Autodesk Inventor part; units mm, degrees
ref_plane "YZ Plane" through (0, 0, 0) normal (1, 0, 0) x (0, 1, 0)
ref_plane "XZ Plane" through (0, 0, 0) normal (0, 1, 0) x (-1, 0, 0)
ref_plane "XY Plane" through (0, 0, 0) normal (0, 0, 1) x (1, 0, 0)
sketch "Sketch1" plane through (0, 0, 0) normal (0, 1, 0) x (-1, 0, 0)
  line L0 (-100, 325) -> (100, 325)
  line L1 (100, 325) -> (100, -325)
  line L2 (100, -325) -> (-100, -325)
  line L3 (-100, -325) -> (-100, 325)
  line L4 (-100, 325) -> (100, -325) construction
  line L5 (100, 325) -> (-100, -325) construction
  point P0 (0, 0)
  dimension "d0" = 200
  dimension "d1" = 650
sketch "Sketch2" plane through (0, 0, 0) normal (0, 1, 0) x (-1, 0, 0)
  point P0 (0, 0)
extrude "Extrusion1" add sketch "Sketch1" along normal blind 20
sketch "Sketch3" plane through (0, 20, 0) normal (0, 1, 0) x (1, 0, 0)
  line L0 (-100, -325) -> (100, -325)
  arc A0 (-100, -325) -> (91.7903, -325) centre (-4.1048, -57.5933) ccw
  point P0 (0, 0)
extrude "Extrusion2" add sketch "Sketch3" against normal blind 20
sketch "Sketch4" plane through (0, 20, 0) normal (0, 1, 0) x (1, 0, 0)
  line L0 (100, 325) -> (-100, 325)
  line L1 (100, 325) -> (36.9346, 362.619)
  line L2 (36.9346, 362.619) -> (0, 367.9885)
  line L3 (0, 367.9885) -> (-39.4325, 362.619)
  line L4 (-39.4325, 362.619) -> (-100, 325)
  point P0 (0, 0)
extrude "Extrusion3" add sketch "Sketch4" against normal blind 20
fillet "Fillet1" radius 2 1 edges at (100, 10, 325)
fillet "Fillet2" radius 4 1 edges at (-100, 10, 325)
chamfer "Chamfer1" distance 2 angle 45 1 edges at (0, 10, -367.9885)
fillet "Fillet3" radius 5 1 edges at (36.9346, 10, -362.619)
fillet "Fillet4" radius 5 1 edges at (-39.4325, 10, -362.619)
sketch "Sketch5" plane through (0, 20, 0) normal (0, 1, 0) x (1, 0, 0)
  line L0 (0, 22.7202) -> (-100, 22.7202)
  line L1 (-100, 325) -> (-100, -322.17)
  line L2 (0, 22.7202) -> (99.1127, 22.7202)
  line L3 (99.1127, 22.7202) -> (-100, 22.7202)
  point P0 (0, 0)
sketch "Sketch6" plane through (0, 20, 0) normal (0, 1, 0) x (1, 0, 0)
  line L0 (93.1857, 273.63) -> (-93.1857, 273.63)
  line L1 (-93.1857, 273.63) -> (-93.1857, 51.0381)
  line L2 (-93.1857, 51.0381) -> (93.1857, 51.0381)
  line L3 (93.1857, 51.0381) -> (93.1857, 273.63)
  line L4 (93.1857, 273.63) -> (-93.1857, 51.0381) construction
  line L5 (-93.1857, 273.63) -> (93.1857, 51.0381) construction
  point P0 (0, 0)
  point P1 (0, 162.334)
extrude "Extrusion4" add sketch "Sketch6" along normal blind 5
sketch "Sketch7" plane through (0, 25, 0) normal (0, 1, 0) x (1, 0, 0)
  line L0 (87.2587, 176.1637) -> (-87.2587, 176.1637)
  line L1 (-87.2587, 176.1637) -> (-87.2587, 57.6236)
  line L2 (-87.2587, 57.6236) -> (87.2587, 57.6236)
  line L3 (87.2587, 57.6236) -> (87.2587, 176.1637)
  line L4 (87.2587, 176.1637) -> (-87.2587, 57.6236) construction
  line L5 (-87.2587, 176.1637) -> (87.2587, 57.6236) construction
  point P0 (0, 0)
  point P1 (0, 116.8937)
extrude "Extrusion5" add sketch "Sketch7" along normal blind 5
sketch "Sketch8" plane through (0, 30, 0) normal (0, 1, 0) x (1, 0, 0)
  circle A0 centre (0, 104.3811) radius 44.0999
  point P0 (0, 0)
extrude "Extrusion6" cut sketch "Sketch8" against normal blind 8
sketch "Sketch9" plane through (0, 30, 0) normal (0, 1, 0) x (1, 0, 0)
  circle A0 centre (-34.3381, 145.486) radius 4.7269
  point P0 (0, 0)
sketch "Sketch10" plane through (0, 0, 0) normal (0, -1, 0) x (1, 0, 0)
  line L0 (100, 323) -> (100, -325)
  line L1 (100, -296.7409) -> (61.6936, -296.7409)
  line L2 (61.6936, -296.7409) -> (61.6936, -172.3341)
  line L3 (61.6936, -172.3341) -> (100, -172.3341)
  line L4 (100, -172.3341) -> (100, -296.7409)
  point P0 (0, 0)
extrude "Extrusion7" cut sketch "Sketch10" against normal blind 15
sketch "Sketch11" plane through (0, 0, 0) normal (0, -1, 0) x (1, 0, 0)
  line L0 (-100, -325) -> (-100, 322.17)
  line L1 (-87.2587, -176.1637) -> (87.2587, -176.1637)
  line L2 (-100, -294.7015) -> (-69.8514, -294.7015)
  line L3 (-69.8514, -294.7015) -> (-69.8514, -176.1637)
  line L4 (-69.8514, -176.1637) -> (-100, -176.1637)
  line L5 (-100, -176.1637) -> (-100, -294.7015)
  point P0 (0, 0)
extrude "Extrusion8" cut sketch "Sketch11" against normal blind 15
sketch "Sketch12" plane through (100, 0, -325) normal (1, 0, 0) x (0, 0, -1)
  circle A0 centre (-575.0278, 0) radius 14.8623
  point P0 (-325, 0)
extrude "Extrusion9" cut sketch "Sketch12" against normal blind 15
sketch "Sketch13" plane through (-100, 0, -325) normal (-1, 0, 0) x (0, 0, 1)
  line L0 (560.1655, 0) -> (589.8902, 0)
  circle A0 centre (575.0278, 0) radius 14.8623
  point P0 (325, 0)
extrude "Extrusion10" cut sketch "Sketch13" against normal blind 15
properties part number "BASE"
The model under review builds one solid part; all positions refer to its coordinate system, in mm. A direction names the side the tool comes from. Round coordinates to 2 decimals unless told otherwise and drop trailing zeros. Loops run counter-clockwise (first coordinate to the right, second up) from the corner with the lowest first, then second, coordinate; pieces in that order, holes last. Notation, with made-up numbers: (1.25, 22) - (45.25, 22) arc R23 cw to (45.25, 47) - close; hole circle Ø6 at (46, 80). An arc over 180 degrees is marked (long way). Use a Markdown table: item, result. Add a question column.
Q1. For probe 1 along Z at (x, y) = (0, 27.25); probe 2 along Y at (x, z) = (1, -124); probe 3 along Z at (x, y) = (72, 14.5), list the stretches that pass through material, from the lowest coordinate up.
Q2. Insertion check: pin 1 Ø12 at (x, y) = (86.5, 8.5) entering from -Z; pin 2 Ø2 at (x, y) = (54, 5) entering from -Z; pin 3 Ø3 at (x, z) = (-73, -216.5) entering from +Y; pin 4 Ø1 at (y, z) = (21, -16) entering from -X. Each pin has a flat end and moves straight along its axis. Give the tip position at first contact, or say it passes through.
Q3. Add section A-A (z = -70.5). State the section outline as (x, y) points.
Q4. Machinability: for faces 1 (the face through (-9.56, 26.06, -61.33)), 2 (the face through (-85, 15, -235)), 3 (the face through (81, 7, -172.334)), which of the approach directions +Z, -Z, +X, -X, +Y, -Y give a long, thin tool a straight path to every point of the face, cutting with its end or side? Answer none if there is none.
Q5. Add section C-C (z = 65). State the section outline as (x, y) points, plus the area to 3 significant figures.
Q6. The part is to be moulded in two halves that separate along X. For faces 4 (the face through (-1, 22, -105)), 5 (the face through (85, 6, 250)), 6 (the face through (81, 7, -296.741)), say which applies: pulls with the +X half, pulls with the -X half, needs draft (parallel to the pull), parting line crosses it, or undercut.
Q7. Add section B-B (x = -19). State the section outline as (y, z) points.
Worked answers:
| question | item | result |
|---|---|---|
| 1 | probe 1 | -176.16 to -148.48, -60.28 to -57.62 |
| 1 | probe 2 | 0 to 22 |
| 1 | probe 3 | -341.7 to -296.74, -172.33 to 331.29 |
| 2 | pin 1 | z = -336.63 |
| 2 | pin 2 | z = -353.04 |
| 2 | pin 3 | y = 25 |
| 2 | pin 4 | through |
| 3 | outline | (-100, 0) - (100, 0) - (100, 20) - (93.19, 20) - (93.19, 25) - (87.26, 25) - (87.26, 30) - (28.23, 30) - (28.23, 22) - (-28.23, 22) - (-28.23, 30) - (-87.26, 30) - (-87.26, 25) - (-93.19, 25) - (-93.19, 20) - (-100, 20) - close |
| 4 | face 1 | +Y |
| 4 | face 2 | -X, -Y |
| 4 | face 3 | +X, -Y |
| 5 | outline | (-100, 0) - (100, 0) - (100, 20) - (-100, 20) - close |
| 5 | area | 4,000 mm² |
| 6 | face 4 | undercut |
| 6 | face 5 | pulls with the +X half |
| 6 | face 6 | needs draft |
| 7 | outline | (0, -365.4) - (20, -365.4) - (20, -273.63) - (25, -273.63) - (25, -176.16) - (30, -176.16) - (30, -144.18) - (22, -144.18) - (22, -64.58) - (30, -64.58) - (30, -57.62) - (25, -57.62) - (25, -51.04) - (20, -51.04) - (20, 341.28) - (0, 341.28) - close |
